```python
from build123d import *

# Parameters (mm, degrees)
F0_R     = 16.5
F0_R_2   = 12.5
F1_DEPTH = 15
F0_R_3   = 10.5
F2_DEPTH = 10
F0_R_4   = 7.5
F3_DEPTH = 12


with BuildPart() as f1:
    # F0 (on Front) → F1 (new body)
    with BuildSketch(Plane.XZ):
        with Locations((-47.357392, 65.085371)):
            Circle(F0_R)
        with Locations((-47.357392, 65.085371)):
            Circle(F0_R_2, mode=Mode.SUBTRACT)
    extrude(amount=F1_DEPTH)

    # F0 (on Front) → F2 (join)
    with BuildSketch(Plane.XZ):
        with BuildLine():
            Line((-25.311984, 74.585371), (-31.190759, 103.385371))
            ThreePointArc((-31.190759, 103.385371), (-47.357392, 116.585371), (-63.524024, 103.385371))
            Line((-63.524024, 103.385371), (-69.402799, 74.585371))
            ThreePointArc((-69.402799, 74.585371), (-71.506721, 65.085371), (-69.402799, 55.585371))
            Line((-69.402799, 55.585371), (-63.524024, 26.785371))
            ThreePointArc((-63.524024, 26.785371), (-47.357392, 13.585371), (-31.190759, 26.785371))
            Line((-31.190759, 26.785371), (-25.311984, 55.585371))
            ThreePointArc((-25.311984, 55.585371), (-23.208062, 65.085371), (-25.311984, 74.585371))
        make_face()
        with Locations((-47.357392, 30.085371)):
            Circle(F0_R_3, mode=Mode.SUBTRACT)
        with Locations((-47.357392, 65.085371)):
            Circle(F0_R, mode=Mode.SUBTRACT)
        with Locations((-47.357392, 100.085371)):
            Circle(F0_R_3, mode=Mode.SUBTRACT)
    extrude(amount=F2_DEPTH)

    # F0 (on Front) → F3 (join)
    with BuildSketch(Plane.XZ):
        with Locations((-47.357392, 100.085371)):
            Circle(F0_R_3)
        with Locations((-47.357392, 100.085371)):
            Circle(F0_R_4, mode=Mode.SUBTRACT)
        with Locations((-47.357392, 30.085371)):
            Circle(F0_R_3)
        with Locations((-47.357392, 30.085371)):
            Circle(F0_R_4, mode=Mode.SUBTRACT)
    extrude(amount=F3_DEPTH)


solid = f1.part
```
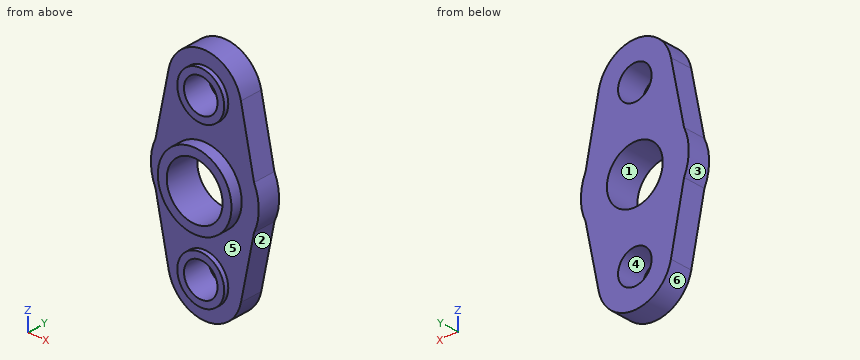
Source: CAD feature listing. Evaluate the final solid. Frame: model axes, mm. Face numbers are marked on the shaded views. A direction names the side the tool comes from. Coordinates: 2 decimals unless noted, no trailing zeros. Write each loop counter-clockwise with the first axis right and the second up, starting at its lowest first coordinate (ties: lowest second). Pieces come first, ordered by that corner, then holes. Notation, with made-up numbers: (48.5, 68.25) - (80.5, 68.25) arc R34 ccw to (80.5, 100.25) - close; hole circle Ø4 at (56.5, -10). An arc over 180 degrees is marked (long way). Answer as a JSON object with one key per item and string values.
Q1. Set-up query: the marked faces 5 and 6. Return all of +Z, -Z, +X, -X, +Y, -Y with unobstructed straight access to the full face (end or side cutting, diameter ignored); none if empty.
Ans:
{"face 5": "-Y", "face 6": "-Z, +Y, -Y"}
Q2. Section query C-C, the plane z = 106.5. Output: boundary loops of the cut face in (x, y).
Ans:
{"outline": "(-62.56, -10) - (-55.67, -10) - (-55.67, -12) - (-51.24, -12) - (-51.24, 0) - (-62.56, 0) - close; (-43.47, -12) - (-39.04, -12) - (-39.04, -10) - (-32.16, -10) - (-32.16, 0) - (-43.47, 0) - close"}
Q3. Section query B-B, the plane x = -51.5. Output: boundary loops of the cut face in (y, z), plus the area to 3 significant figures.
Ans:
{"outline": "(-15, 49.11) - (-10, 49.11) - (-10, 39.73) - (-12, 39.73) - (-12, 36.34) - (0, 36.34) - (0, 53.29) - (-15, 53.29) - close; (-15, 76.88) - (0, 76.88) - (0, 93.83) - (-12, 93.83) - (-12, 90.44) - (-10, 90.44) - (-10, 81.06) - (-15, 81.06) - close; (-12, 20.44) - (-10, 20.44) - (-10, 14.11) - (0, 14.11) - (0, 23.83) - (-12, 23.83) - close; (-12, 106.34) - (0, 106.34) - (0, 116.06) - (-10, 116.06) - (-10, 109.73) - (-12, 109.73) - close", "area": "602 mm2"}
Q4. Material intervals for line 1 (Z direction, x = -44.5, y = -1); line 2 (Z direction, x = -48, y = -0.75); line 3 (Y direction, x = -59, z = 52.5), sorted ascending. Write a range as [from, to].
Ans:
{"line 1": "z = [13.83, 23.15], [37.02, 52.92], [77.25, 93.15], [107.02, 116.34]", "line 2": "z = [13.6, 22.61], [37.56, 52.6], [77.57, 92.61], [107.56, 116.57]", "line 3": "y = [-10, 0]"}
Q5. Draft query along X for the marked faces 1, 2, 3 and 4. Return one class per face: released by +X, released by -X, zero draft, split by the parting line, or undercut.
Ans:
{"face 1": "undercut", "face 2": "released by +X", "face 3": "released by -X", "face 4": "undercut"}
Q6. Section query A-A, the plane y = -11. Output: boundary loops of the cut face in (x, z), plus the area to 3 significant figures.
Ans:
{"outline": "circle Ø33 at (-47.36, 65.09); circle Ø21 at (-47.36, 30.09); circle Ø21 at (-47.36, 100.09); hole circle Ø25 at (-47.36, 65.09); hole circle Ø15 at (-47.36, 30.09); hole circle Ø15 at (-47.36, 100.09)", "area": "704 mm2"}
Q7. First-contact query: pin 1 Ø23 at (x, z) = (-46.5, 100.5) entering from -Y; pin 2 Ø1 at (x, y) = (-45.5, -2) entering from +Z; pin 3 Ø6 at (x, z) = (-29, 46.5) entering from +Y; pin 4 Ø1.5 at (y, z) = (-10.5, 31) entering from +X. Flat tips, straight axial feed; report the tip coordinate or a pass-through.
Ans:
{"pin 1": "stops at y = -12", "pin 2": "stops at z = 116.53", "pin 3": "stops at y = 0", "pin 4": "stops at x = -30.22"}
Q8. Section query D-D, the plane y = -1. Output: boundary loops of the cut face in (x, z).
Ans:
{"outline": "(-69.4, 55.59) - (-63.52, 26.79) arc R16.5 ccw to (-31.19, 26.79) - (-25.31, 55.59) arc R22.5 ccw to (-25.31, 74.59) - (-31.19, 103.39) arc R16.5 ccw to (-63.52, 103.39) - (-69.4, 74.59) arc R22.5 ccw to start; hole circle Ø25 at (-47.36, 65.09); hole circle Ø15 at (-47.36, 30.09); hole circle Ø15 at (-47.36, 100.09)"}
